Can you work these out from the model? Positions are in its coordinate system, mm. A direction names the side the tool comes from. Round coordinates to 2 decimals unless told otherwise and drop trailing zeros. Loops run counter-clockwise (first coordinate to the right, second up) from the corner with the lowest first, then second, coordinate; pieces in that order, holes last.
```python
from build123d import *
from build123d import SkipClean  # not in build123d's __all__

# Parameters (mm, degrees)
F0_R     = 20
F0_R_2   = 10
F1_DEPTH = 5
F3_DEPTH = 5


with BuildPart() as f1:
    # F0 (on Top) → F1 (new body)
    with BuildSketch(Plane.XY):
        Circle(F0_R)
        Circle(F0_R_2, mode=Mode.SUBTRACT)
    extrude(amount=F1_DEPTH)

    # F2 (on face) → F3 (join)
    with BuildSketch(Plane.XY.offset(5)):
        with BuildLine():
            ThreePointArc((-5, -8.6602540378), (-7.0062926922, -7.1352549156), (-8.5676274578, -5.1571076917))
            Line((-8.5676274578, -5.1571076917), (-17.1352549156, -10.3142153835))
            ThreePointArc((-17.1352549156, -10.3142153835), (-14.0125853844, -14.2705098312), (-10, -17.3205080757))
            Line((-10, -17.3205080757), (-5, -8.6602540378))
        make_face()
        with BuildLine():
            ThreePointArc((10, 0), (9.6824583655, -2.5), (8.75, -4.8412291828))
            Line((8.75, -4.8412291828), (17.5, -9.6824583655))
            ThreePointArc((17.5, -9.6824583655), (19.364916731, -5), (20, 0))
            Line((20, 0), (10, 0))
        make_face()
        with BuildLine():
            ThreePointArc((-5, 8.6602540378), (-2.6761656733, 9.6352549156), (-0.1823725422, 9.9983368745))
            Line((-0.1823725422, 9.9983368745), (-0.3647450844, 19.996673749))
            ThreePointArc((-0.3647450844, 19.996673749), (-5.3523313466, 19.2705098312), (-10, 17.3205080757))
            Line((-10, 17.3205080757), (-5, 8.6602540378))
        make_face()
    with SkipClean():  # cleaning this boolean's faces spoils the solid; the shape is the same uncleaned
        extrude(amount=F3_DEPTH)


solid = f1.part
```
(1) Which directions (+Z, -Z, +X, -X, +Y, -Y) give clear straight access to the entire face, cutting with the end or side of a thin tool? Please do faces 5 (the flat face through (-12.79, -7.7, 7.46)), 6 (the flat face through (15, 0, 7)), 7 (the flat face through (10, 10, 5)).
(2) We'd pull the mould along X, two halves only. Please class faces 1 (the flat face through (13.064, -7.228, 7.465)), 2 (the flat face through (-7.535, 13.051, 7.465)), 3 (the flat face through (4, -14, 5)), 4 (the flat face through (-13, 4, 5)): released by +X, released by -X, zero draft, split by the parting line, or undercut.
(3) Suppose I cut it at D-D (x = -11.5). Write out the boundary of the cut face in (y, z), then the cut area to 3 significant figures.
(4) For pin 1 (1.5 mm diameter, centred on x = 3.5, y = 11, fed in from +Z); pin 2 (6 mm diameter, centred on x = 9, y = 12.5, fed in from -Z); pin 3 (1 mm diameter, centred on x = 14, z = 8, fed in from +Y), each with a flat end and sliding along its axis, tell me the tip position at first contact or that it passes through.
(5) If I drill on line 1 (Y direction, x = 0, z = 3.7); line 2 (Z direction, x = 1.5, y = 14), over which ranges is the centre line in solid material (lowest first)?
(6) Suppose I cut it at C-C (x = 5.5). Write out the boundary of the cut face in (y, z), then the cut area to 3 significant figures.
(7) Suppose I cut it at B-B (z = 6.25). Write out the boundary of the cut face in (x, y).
(8) Suppose I cut it at A-A (y = 4). Write out the boundary of the cut face in (x, z).
Check result:
1. face 5: +Z, -X
1. face 6: +Z, +X, -X, +Y
1. face 7: +Z, +X, +Y
2. face 1: undercut
2. face 2: released by -X
2. face 3: undercut
2. face 4: zero draft
3. outline: (-16.36, 0) - (16.36, 0) - (16.36, 5) - (-6.92, 5) - (-6.92, 10) - (-16.36, 10) - close
3. area: 211 mm2
4. pin 1: stops at z = 5
4. pin 2: stops at z = 0
4. pin 3: stops at y = 0
5. line 1: y = -20 to -10, 10 to 20
5. line 2: z = 0 to 5
6. outline: (-19.23, 0) - (-8.35, 0) - (-8.35, 5) - (-19.23, 5) - close; (8.35, 0) - (19.23, 0) - (19.23, 5) - (8.35, 5) - close
6. area: 109 mm2
7. outline: (-17.14, -10.31) arc R20 ccw to (-10, -17.32) - (-5, -8.66) arc R10 cw to (-8.57, -5.16) - close; (-10, 17.32) - (-5, 8.66) arc R10 cw to (-0.18, 10) - (-0.36, 20) arc R20 ccw to start; (8.75, -4.84) - (17.5, -9.68) arc R20 ccw to (20, 0) - (10, 0) arc R10 cw to start
8. outline: (-19.6, 0) - (-9.17, 0) - (-9.17, 5) - (-19.6, 5) - close; (9.17, 0) - (19.6, 0) - (19.6, 5) - (9.17, 5) - close
